Here's how the part is built. I have some questions about the finished solid (model axes, mm). Give positions to 0.01 mm unless a question says otherwise; leave off trailing zeros. Loops run counter-clockwise (first coordinate to the right, second up) from the corner with the lowest first, then second, coordinate; pieces in that order, holes last. Notation, with made-up numbers: (46, 70.25) - (71, 70.25) arc R24 ccw to (71, 101.25) - close; hole circle Ø11 at (-36, 68). An arc over 180 degrees is marked (long way). Use a Markdown table: item, result.
from build123d import *

# Parameters (mm, degrees)
SKETCH2_W           = 255
SKETCH2_H           = 65
BOSS_EXTRUDE1_DEPTH = 5
SKETCH3_W           = 6
SKETCH3_H           = 65
BOSS_EXTRUDE2_DEPTH = 5
SKETCH3_3_W         = 5
SKETCH3_3_H         = 30
CUT_EXTRUDE1_DEPTH  = 10
SKETCH4_W           = 6
SKETCH4_H           = 65
CUT_EXTRUDE2_DEPTH  = 10
SKETCH6_W           = 255
SKETCH6_H           = 5
BOSS_EXTRUDE3_DEPTH = 185
CUT_EXTRUDE3_DEPTH  = 185
SKETCH9_R           = 1.5
CUT_EXTRUDE4_DEPTH  = 185
SKETCH10_R          = 1.5
CUT_EXTRUDE5_DEPTH  = 185
SKETCH11_R          = 2
CUT_EXTRUDE6_DEPTH  = 10


with BuildPart() as part:
    # Sketch2 → Boss-Extrude1 (new body)
    with BuildSketch(Plane(origin=(0, 0, 0), x_dir=(1, 0, 0), z_dir=(0, 1, 0))):
        with Locations((127.5, 32.5)):
            Rectangle(SKETCH2_W, SKETCH2_H)
    extrude(amount=BOSS_EXTRUDE1_DEPTH)

    # Sketch3 → Boss-Extrude2 (add)
    with BuildSketch(Plane(origin=(0, 5, 0), x_dir=(1, 0, 0), z_dir=(0, 1, 0))):
        Polygon((261, 65), (255, 65), (255, 47.5), (255, 17.5), (255, 0), (261, 0), align=None)
        with Locations((-3, 32.5)):
            Rectangle(SKETCH3_W, SKETCH3_H)
    extrude(amount=-BOSS_EXTRUDE2_DEPTH)

    # Sketch3<3> → Cut-Extrude1 (cut)
    with BuildSketch(Plane(origin=(0, 5, 0), x_dir=(1, 0, 0), z_dir=(0, 1, 0))):
        with Locations((252.5, 32.5)):
            Rectangle(SKETCH3_3_W, SKETCH3_3_H)
        with Locations((2.5, 32.5)):
            Rectangle(SKETCH3_3_W, SKETCH3_3_H)
    extrude(amount=-CUT_EXTRUDE1_DEPTH, mode=Mode.SUBTRACT)

    # Sketch4 → Cut-Extrude2 (cut)
    with BuildSketch(Plane.XZ):
        Polygon((255, -47.5), (255, -65), (261, -65), (261, 0), (255, 0), align=None)
        with Locations((-3, -32.5)):
            Rectangle(SKETCH4_W, SKETCH4_H)
    extrude(amount=-CUT_EXTRUDE2_DEPTH, mode=Mode.SUBTRACT)

    # Sketch6 → Boss-Extrude3 (add)
    with BuildSketch(Plane.XY):
        with Locations((127.5, 2.5)):
            Rectangle(SKETCH6_W, SKETCH6_H)
    extrude(amount=BOSS_EXTRUDE3_DEPTH)

    # Sketch8 → Cut-Extrude3 (cut)
    with BuildSketch(Plane(origin=(0, 5, 0), x_dir=(1, 0, 0), z_dir=(0, 1, 0))):
        Polygon((127.5, -185), (191.25, -185), (191.25, -180), (127.5, -180), (63.75, -180), (63.75, -185), align=None)
    extrude(amount=-CUT_EXTRUDE3_DEPTH, mode=Mode.SUBTRACT)

    # Sketch9 → Cut-Extrude4 (cut)
    with BuildSketch(Plane(origin=(0, 5, 0), x_dir=(1, 0, 0), z_dir=(0, 1, 0))):
        with Locations((223.125, -170)):
            Circle(SKETCH9_R)
        with Locations((31.875, -170)):
            Circle(SKETCH9_R)
    extrude(amount=-CUT_EXTRUDE4_DEPTH, mode=Mode.SUBTRACT)

    # Sketch10 → Cut-Extrude5 (cut)
    with BuildSketch(Plane(origin=(0, 5, 0), x_dir=(1, 0, 0), z_dir=(0, 1, 0))):
        with Locations((240, 8.75)):
            Circle(SKETCH10_R)
        with Locations((15, 8.75)):
            Circle(SKETCH10_R)
    extrude(amount=-CUT_EXTRUDE5_DEPTH, mode=Mode.SUBTRACT)

    # Sketch11 → Cut-Extrude6 (cut)
    with BuildSketch(Plane(origin=(0, 5, 0), x_dir=(1, 0, 0), z_dir=(0, 1, 0))):
        with Locations((240, 8.75)):
            Circle(SKETCH11_R)
        with Locations((15, 8.75)):
            Circle(SKETCH11_R)
        with Locations((31.875, -170)):
            Circle(SKETCH11_R)
        with Locations((223.125, -170)):
            Circle(SKETCH11_R)
    extrude(amount=-CUT_EXTRUDE6_DEPTH, mode=Mode.SUBTRACT)


solid = part.part
(1) Suppose I cut it at B-B on x = 140.5. Write out the boundary of the cut face in (y, z), plus the area to 4 significant figures.
A:
| item | result |
|---|---|
| outline | (0, -65) - (5, -65) - (5, 180) - (0, 180) - close |
| area | 1,225 mm2 |
(2) Will these pins go through, and if not, where does the flat tip stop? pin 1 (6.5 mm diameter, centred on x = 240, z = -8.75, fed in from -Y); pin 2 (1.5 mm diameter, centred on y = 3.5, z = -28.5, fed in from -X); pin 3 (2.5 mm diameter, centred on y = 2.5, z = -27.5, fed in from +X).
A:
| item | result |
|---|---|
| pin 1 | y = 0 |
| pin 2 | x = 5 |
| pin 3 | x = 250 |
(3) If I drill on line 1 (X direction, y = 3.05, z = 170) (3 decimals); line 2 (X direction, y = 2.25, z = -8.75); line 3 (Z direction, x = 240, y = 2.7), over which ranges is the centre line in solid material (lowest first)?
A:
| item | result |
|---|---|
| line 1 | 0 to 29.875, 33.875 to 221.125, 225.125 to 255 |
| line 2 | 0 to 13, 17 to 238, 242 to 255 |
| line 3 | -65 to -10.75, -6.75 to 185 |
(4) Suppose I cut it at A-A on y = 4.25. Write out the boundary of the cut face in (x, z) (3 decimals).
A:
| item | result |
|---|---|
| outline | (0, -65) - (255, -65) - (255, -47.5) - (250, -47.5) - (250, -17.5) - (255, -17.5) - (255, 185) - (191.25, 185) - (191.25, 180) - (63.75, 180) - (63.75, 185) - (0, 185) - (0, -17.5) - (5, -17.5) - (5, -47.5) - (0, -47.5) - close; hole circle Ø4 at (15, -8.75); hole circle Ø4 at (31.875, 170); hole circle Ø4 at (223.125, 170); hole circle Ø4 at (240, -8.75) |
